Design review of the part built by this model. Coordinates are the model's own, in mm. Face numbers are marked on the shaded views. A direction names the side the tool comes from. Coordinates: 2 decimals unless noted, no trailing zeros. Answer as a JSON object with one key per item and string values.
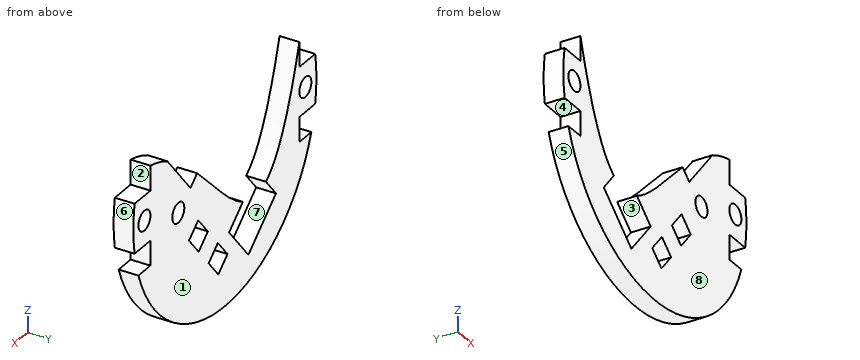
```python
from build123d import *

# Parameters (mm, degrees)
CROQUIS1_R              = 30.5
SALIENTE_EXTRUIR1_DEPTH = 4
CROQUIS2_R              = 2
CORTAR_EXTRUIR1_DEPTH   = 4
CORTAR_EXTRUIR3_START   = -4
CORTAR_EXTRUIR3_DEPTH   = 4
CORTAR_EXTRUIR5_START   = -4
CROQUIS7_R              = 2
CORTAR_EXTRUIR5_DEPTH   = 4
CORTAR_EXTRUIR6_DEPTH   = 10
CROQUIS10_R             = 2
CORTAR_EXTRUIR7_DEPTH   = 4


with BuildPart() as part:
    # Croquis1 → Saliente-Extruir1 (new body)
    with BuildSketch(Plane(origin=(0, 0, 0), x_dir=(1, 0, 0), z_dir=(0, 1, 0))):
        with Locations(Location((0, 0, 0), (0, 0, 270))):
            Circle(CROQUIS1_R)
    extrude(amount=SALIENTE_EXTRUIR1_DEPTH)

    # Croquis2 → Cortar-Extruir1 (cut)
    with BuildSketch(Plane(origin=(0, 4, 0), x_dir=(1, 0, 0), z_dir=(0, 1, 0))):
        with Locations(Location((0, 0, 0), (0, 0, 270))):
            Circle(CROQUIS2_R)
    extrude(amount=-CORTAR_EXTRUIR1_DEPTH, mode=Mode.SUBTRACT)

    # Croquis5 → Cortar-Extruir3 (cut)
    with BuildSketch(Plane(origin=(0, 4, 0), x_dir=(1, 0, 0), z_dir=(0, 1, 0)).offset(CORTAR_EXTRUIR3_START)):
        with BuildLine():
            Line((28.814059068, 5), (30.087372767, 5))
            ThreePointArc((30.087372767, 5), (29.556634924, 7.526973624), (28.814059068, 10))
            Line((28.814059068, 10), (24.814059068, 10))
            Line((24.814059068, 10), (24.814059068, 5))
            Line((24.814059068, 5), (28.814059068, 5))
        make_face()
        with BuildLine():
            Line((30.087372767, -5), (28.814059068, -5))
            Line((28.814059068, -5), (24.814059068, -5))
            Line((24.814059068, -5), (24.814059068, -10))
            Line((24.814059068, -10), (28.814059068, -10))
            ThreePointArc((28.814059068, -10), (29.556634924, -7.526973624), (30.087372767, -5))
        make_face()
        with BuildLine():
            Line((-24.814059068, 5), (-24.814059068, 10))
            Line((-24.814059068, 10), (-28.814059068, 10))
            ThreePointArc((-28.814059068, 10), (-29.556634924, 7.526973624), (-30.087372767, 5))
            Line((-30.087372767, 5), (-28.814059068, 5))
            Line((-28.814059068, 5), (-24.814059068, 5))
        make_face()
        with BuildLine():
            Line((-28.814059068, -10), (-24.814059068, -10))
            Line((-24.814059068, -10), (-24.814059068, -5))
            Line((-24.814059068, -5), (-28.814059068, -5))
            Line((-28.814059068, -5), (-30.087372767, -5))
            ThreePointArc((-30.087372767, -5), (-29.556634924, -7.526973624), (-28.814059068, -10))
        make_face()
    extrude(amount=CORTAR_EXTRUIR3_DEPTH, mode=Mode.SUBTRACT)

    # Croquis7 → Cortar-Extruir5 (cut)
    with BuildSketch(Plane(origin=(0, 4, 0), x_dir=(1, 0, 0), z_dir=(0, 1, 0)).offset(CORTAR_EXTRUIR5_START)):
        with Locations(Location((15.526809242, 4.053864794, 0), (0, 0, 270))):
            Circle(CROQUIS7_R)
        Polygon((2.194434654, 23.054217761), (-0.869743118, 20.483067322), (2.34419493, 16.652845106), (5.408372702, 19.223995545), align=None)
        with BuildLine():
            Line((-24.814059068, -10), (-28.814059068, -10))
            ThreePointArc((-28.814059068, -10), (0, -30.5), (28.814059068, -10))
            Line((28.814059068, -10), (24.814059068, -10))
            add(Edge.make_bspline(
                [(24.814059068, -10), (22.863263717, -9.657344338), (20.984021298, -8.980450277), (19.168992989, -8.065339906)],
                knots=[0, 0, 0, 0, 0.087850084, 0.087850084, 0.087850084, 0.087850084], degree=3))
            Line((19.168992989, -8.065339906), (11.455541673, 1.127193412))
            Line((11.455541673, 1.127193412), (9.248678515, -0.72458465))
            add(Edge.make_bspline(
                [(9.248678515, -0.72458465), (3.657558626, 4.465361799), (-1.318373357, 10.288134416), (-5.99647718, 12.591356616)],
                knots=[0.258799312, 0.258799312, 0.258799312, 0.258799312, 0.567154107, 0.567154107, 0.567154107, 0.567154107], degree=3))
            Line((-5.99647718, 12.591356616), (-1.400210521, 16.448082274))
            Line((-1.400210521, 16.448082274), (-7.828086618, 24.108526705))
            Line((-7.828086618, 24.108526705), (-17.020619935, 16.395075389))
            Line((-17.020619935, 16.395075389), (-13.66601447, 12.397212273))
            add(Edge.make_bspline(
                [(-13.66601447, 12.397212273), (-17.403465693, 9.897923685), (-21.056529869, 3.255841362), (-24.814059068, -10)],
                knots=[0.740637404, 0.740637404, 0.740637404, 0.740637404, 1, 1, 1, 1], degree=3))
        make_face()
    extrude(amount=CORTAR_EXTRUIR5_DEPTH, mode=Mode.SUBTRACT)

    # Croquis9 → Cortar-Extruir6 (cut)
    with BuildSketch(Plane(origin=(0, 4, 0), x_dir=(1, 0, 0), z_dir=(0, 1, 0))):
        Polygon((8.737462625, 15.25654067), (5.673284852, 12.685390231), (8.887222901, 8.855168016), (11.951400673, 11.426318455), align=None)
    extrude(amount=-CORTAR_EXTRUIR6_DEPTH, mode=Mode.SUBTRACT)

    # Croquis10 → Cortar-Extruir7 (cut)
    with BuildSketch(Plane(origin=(0, 4, 0), x_dir=(1, 0, 0), z_dir=(0, 1, 0))):
        with Locations(Location((-26.814059068, 0, 0), (0, 0, 270))):
            Circle(CROQUIS10_R)
        with Locations(Location((26.814059068, 0, 0), (0, 0, 270))):
            Circle(CROQUIS10_R)
    extrude(amount=-CORTAR_EXTRUIR7_DEPTH, mode=Mode.SUBTRACT)


solid = part.part
```
(1) Take a section at A-A, the plane y = 2.7. Give the number of separate pieces and of enclosed holes in the cut face, and give its area (3 significant figures).
Solved:
{"separate pieces": "1", "enclosed holes": "5", "area": "1,130 mm^2"}
(2) Tool access review of the marked faces 1, 2, 3, 4 and 5: name each direction out of +Z, -Z, +X, -X, +Y, -Y from which nothing blocks a thin tool from reaching the whole face with its end or side.
Solved:
{"face 1": "+Z, -Z, +X, -X, +Y", "face 2": "+Z, +X, +Y, -Y", "face 3": "+Y, -Y", "face 4": "-X, +Y, -Y", "face 5": "-Z, +Y, -Y"}
(3) The part is to be moulded in two halves that separate along Z. For the marked faces 6, 7 and 8, say which applies: pulls with the +Z half, pulls with the -Z half, needs draft (parallel to the pull), parting line crosses it, or undercut.
Solved:
{"face 6": "parting line crosses it", "face 7": "undercut", "face 8": "needs draft"}
(4) To check wall thickness, follow line 1 (X direction, y = 0.25, z = -22.5); line 2 (X direction, y = 3.5, z = -14.5); line 3 (X direction, y = 1.3, z = 0). State the ranges of each line that lie inside material, in increasing order. Write a range as from..to.
Solved:
{"line 1": "x = -20.59..-9.75, -6.48..1.53, 2.66..20.59", "line 2": "x = -26.83..-15.43, -3.72..7.84, 9.37..26.83", "line 3": "x = -30.5..-28.81, -24.81..-21.54, 8.48..10.11, 12.4..24.81, 28.81..30.5"}
(5) For pin 1 (1.2 mm diameter, centred on y = 2, z = 6.5, fed in from +X); pin 2 (2 mm diameter, centred on x = -27, y = 1, fed in from +Z); pin 3 (2 mm diameter, centred on x = 28.5, y = 2, fed in from -Z), all flat-tipped, find the tip position at first contact; note any pin that passes through.
Solved:
{"pin 1": "stops at x = 24.81", "pin 2": "stops at z = 5", "pin 3": "stops at z = -13.19"}
